Geometry check sheet. Reference: the model listing, model coordinates, mm. Face numbers are marked on the shaded views. A direction names the side the tool comes from. Give positions to 0.01 mm unless a question says otherwise; leave off trailing zeros. Loops run counter-clockwise (first coordinate to the right, second up) from the corner with the lowest first, then second, coordinate; pieces in that order, holes last.
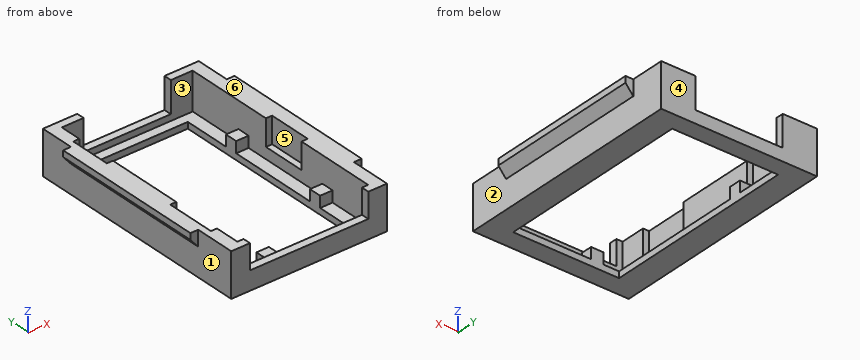
```python
from build123d import *

# Parameters (mm, degrees)
F0_W      = 25
F0_H      = 38
F1_DEPTH  = 7
F2_W      = 21
F2_H      = 34.5
F3_DEPTH  = 6
F4_W      = 2
F4_H      = 2
F5_DEPTH  = 1.8
F6_W      = 17
F6_H      = 31.25
F7_DEPTH  = 7.001
F8_W      = 0.0254269466
F8_H      = 6.6
F8_W_2    = 0.9745730534
F8_W_3    = 1
F8_H_2    = 7
F8_H_3    = 8
F9_DEPTH  = 4.2
F11_W     = 14
F11_H     = 5
F12_DEPTH = 5
F13_DEPTH = 1
F15_DEPTH = 12.5
F16_W     = 19
F16_H     = 4
F17_DEPTH = 3


# Not quite as in the source:
# - a pattern or mirror of a feature is missing from the dataset's text; its kind, count and spacing are read off the source's solid
# - a feature names something its author has since deleted; it is built from what else it names


with BuildPart() as f1:
    # F0 (on Top) → F1 (new body)
    with BuildSketch(Plane.XY):
        Rectangle(F0_W, F0_H)
    extrude(amount=F1_DEPTH)

    # F2 (on face) → F3 (cut)
    with BuildSketch(Plane.XY.offset(7)):
        with Locations((0, -0.5)):
            Rectangle(F2_W, F2_H)
    extrude(amount=-F3_DEPTH, mode=Mode.SUBTRACT)

    # F4 (on face) → F5 (join)
    with BuildSketch(Plane.XY.offset(1)):
        with Locations((-9.5, 6.75)):
            Rectangle(F4_W, F4_H)
        with Locations((9.5, 6.75)):
            Rectangle(F4_W, F4_H)
        with Locations((9.5, -9.75)):
            Rectangle(F4_W, F4_H)
        with Locations((-5, -17)):
            Rectangle(F4_W, F4_H)
    extrude(amount=F5_DEPTH)

    # F6 (on Top) → F7 (cut, through all)
    with BuildSketch(Plane.XY):
        with Locations((0, -0.375)):
            Rectangle(F6_W, F6_H)
    extrude(amount=F7_DEPTH, mode=Mode.SUBTRACT)

    # F8 (on face) → F9 (cut, through all)
    with BuildSketch(Plane.XY.offset(7)):
        with Locations((-10.4872865267, 10.0065428064)):
            Rectangle(F8_W, F8_H)
        with Locations((-10.9872865267, 10.0065428064)):
            Rectangle(F8_W_2, F8_H)
        with Locations((11, -1.15)):
            Rectangle(F8_W_3, F8_H_2)
        with Locations((-10.9872865267, -9.75)):
            Rectangle(F8_W_2, F8_H_3)
    extrude(amount=-F9_DEPTH, mode=Mode.SUBTRACT)

    # F11 (on offset) → F12 (cut)
    with BuildSketch(Plane.XY.offset(2)):
        with Locations((0, 19.25)):
            Rectangle(F11_W, F11_H)
    extrude(amount=F12_DEPTH, mode=Mode.SUBTRACT)

    # F13 (cut): a face of the model
    f13_faces = [f1.faces().sort_by_distance(p)[0] for p in [
        (0, 19, 0.2596150997),
    ]]
    extrude(f13_faces, amount=-F13_DEPTH, mode=Mode.SUBTRACT)

    # F14 (on Front) → F15 (join, symmetric)
    with BuildSketch(Plane.XZ):
        Polygon((13.75, 7), (12.5, 7), (12.5, 4.5103080093), (13.75, 6), align=None)
    f15 = extrude(amount=F15_DEPTH, both=True)

    # F15_copies: F15 across plane
    add(f15.mirror(Plane(origin=(0, 0, 0), x_dir=(0, 0, -1), z_dir=(-1, 0, 0))))

    # F16 (on face) → F17 (cut)
    with BuildSketch(Plane.XZ.offset(19)):
        with Locations((0, 5)):
            Rectangle(F16_W, F16_H)
    extrude(amount=-F17_DEPTH, mode=Mode.SUBTRACT)


solid = f1.part
```
1) Sectioned sample at B-B on z = 3.5. Enter the section's corners in (x, y).
2) Depth check by flat-ended pin: P1, Ø5, axis at x = -5.5, y = 3, coming from the +Z side; P2, Ø2, axis at x = -2.5, z = 3.5, coming from the +Y side; P3, Ø1.4, axis at y = -18.5, z = 5.5, coming from the +X side; P4, Ø1.9, axis at x = -5, y = -17, coming from the +Z side. Enter the tip coordinate at first touch or a pass-through.
3) Tool access check on the marked faces 5 and 6. Record the directions out of +Z, -Z, +X, -X, +Y, -Y that give a thin tool (end or side, any length) a straight path to the whole face; none if there is none.
4) Sectioned sample at D-D on z = 0.5. Enter the section's corners in (x, y).
5) Sectioned sample at A-A on y = -7. Enter the section's corners in (x, z), plus the area to 3 significant figures.
6) Sectioned sample at C-C on x = 7.75. Enter the section's corners in (y, z).
7) Mould release check, pull along X, two halves, no side actions. Record for the marked faces 1, 2, 3 and 4: +X half, -X half, draft (parallel to the pull), parting line (faces both ways), or undercut.
8) Scan lines: line 1 along X through (y, z) = (11.5, 2.25); line 2 along Y through (x, z) = (-4.5, 0.5); line 3 along X through (y, z) = (5, 6.5). Record each from-to range of solid material in increasing order.
Determined:
1. outline: (-12.5, -19) - (-9.5, -19) - (-9.5, -17.75) - (-10.5, -17.75) - (-10.5, -13.75) - (-11.47, -13.75) - (-11.47, -5.75) - (-10.5, -5.75) - (-10.5, 6.71) - (-11.47, 6.71) - (-11.47, 13.31) - (-10.5, 13.31) - (-10.5, 16.75) - (-7, 16.75) - (-7, 18) - (-12.5, 18) - close; (7, 16.75) - (10.5, 16.75) - (10.5, 2.35) - (11.5, 2.35) - (11.5, -4.65) - (10.5, -4.65) - (10.5, -17.75) - (9.5, -17.75) - (9.5, -19) - (12.5, -19) - (12.5, 18) - (7, 18) - close
2. P1: passes through
2. P2: stops at y = -17.75
2. P3: stops at x = 12.5
2. P4: stops at z = 3
3. face 5: +Z
3. face 6: +Z, +X, -X, +Y, -Y
4. outline: (-12.5, -19) - (12.5, -19) - (12.5, 18) - (-12.5, 18) - close; hole (-8.5, -16) - (8.5, -16) - (8.5, 15.25) - (-8.5, 15.25) - close
5. outline: (-13.75, 6) - (-12.5, 4.51) - (-12.5, 0) - (-8.5, 0) - (-8.5, 1) - (-10.5, 1) - (-10.5, 2.8) - (-11.47, 2.8) - (-11.47, 7) - (-13.75, 7) - close; (8.5, 0) - (12.5, 0) - (12.5, 4.51) - (13.75, 6) - (13.75, 7) - (10.5, 7) - (10.5, 1) - (8.5, 1) - close
5. area: 32.3 mm2
6. outline: (-19, 0) - (-16, 0) - (-16, 1) - (-17.75, 1) - (-17.75, 3) - (-19, 3) - close; (15.25, 0) - (18, 0) - (18, 7) - (16.75, 7) - (16.75, 1) - (15.25, 1) - close
7. face 1: -X half
7. face 2: +X half
7. face 3: undercut
7. face 4: draft
8. line 1: x = -12.5 to -10.5, 10.5 to 12.5
8. line 2: y = -19 to -16, 15.25 to 18
8. line 3: x = -13.75 to -10.5, 10.5 to 13.75
